from build123d import *

# Parameters (mm, degrees)
ESQUISSE1_R        = 1.5
BOSS_EXTRU_1_DEPTH = 5
BOSS_EXTRU_2_DEPTH = 20


with BuildPart() as part:
    # Esquisse1 → Boss.-Extru.1 (new body)
    with BuildSketch(Plane.XY):
        with BuildLine():
            Line((2.411392109, 3.191424149), (-33.53228234, 30.349924212))
            ThreePointArc((-33.53228234, 30.349924212), (-39.142258528, 29.531111427), (-38.389494778, 23.911891379))
            Line((-38.389494778, 23.911891379), (-2.406799918, -3.194888755))
            ThreePointArc((-2.406799918, -3.194888755), (3.193157277, -2.409096636), (2.411392109, 3.191424149))
        make_face()
        with Locations((-35.923019369, 27.102337158)):
            Circle(ESQUISSE1_R, mode=Mode.SUBTRACT)
        Circle(ESQUISSE1_R, mode=Mode.SUBTRACT)
    boss_extru_1 = extrude(amount=BOSS_EXTRU_1_DEPTH)

    # Esquisse2 → Boss.-Extru.2 (add)
    with BuildSketch(Plane(origin=(0, 0, 0), x_dir=(-1, 0, 0), z_dir=(0, 0, -1))):
        Polygon((20.560906603, 20.548947707), (25.40403733, 14.129579595), (29.397447291, 17.137928086), (24.549986024, 23.563036149), align=None)
    boss_extru_2 = extrude(amount=BOSS_EXTRU_2_DEPTH)

    # Symétrie1: Boss.-Extru.1, Boss.-Extru.2 across plane
    add(boss_extru_1.mirror(Plane.XY.offset(-20)))
    add(boss_extru_2.mirror(Plane.XY.offset(-20)))


solid = part.part
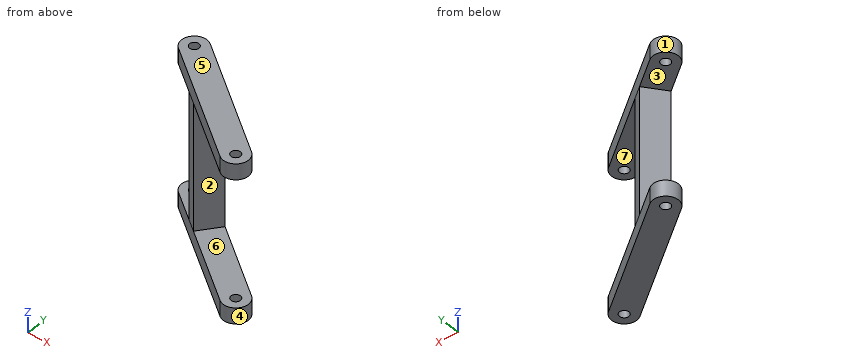
Read the model definition and answer for the solid it produces. Units are mm, in the model's axes. Face numbers are marked on the shaded views. A direction names the side the tool comes from. Coordinates: 2 decimals unless noted, no trailing zeros. Order: outer loops, then holes, each group sorted by start corner. A loop starts at its lowest first (then second) coordinate and runs counter-clockwise, first axis right, second up. Notation, with made-up numbers: (22.25, -13) -> (38.25, -13) arc R25 cw to (38.25, 9) -> close; hole circle Ø1 at (75, -40). An arc over 180 degrees is marked (long way). Answer as a JSON object with one key per item and string values.
1) Consider line 1 along Z through (x, y) = (-4, 8); line 2 along X through (y, z) = (17.5, -34.5); line 3 along Y through (x, z) = (-22.5, -39.5). Determine where each line is inside the solid, lowest interval first. Write a range as from..to.
Model answer:
{"line 1": "z = -45..-40, 0..5", "line 2": "x = -29.12..-22.86", "line 3": "y = 17.98..22.01"}
2) The mould has two halves that part along Z. Classify the marked faces 4, 5, 6 and 7: released by +Z, released by -Z, zero draft, split by the parting line, or undercut.
Model answer:
{"face 4": "zero draft", "face 5": "released by +Z", "face 6": "undercut", "face 7": "undercut"}
3) A cutting plane is placed at C-C, the plane x = -10.5. Determine the outline of the cut face in (y, z), plus the area to 3 significant figures.
Model answer:
{"outline": "(2.9, -45) -> (12.95, -45) -> (12.95, -40) -> (2.9, -40) -> close; (2.9, 0) -> (12.95, 0) -> (12.95, 5) -> (2.9, 5) -> close", "area": "100 mm²"}
4) This flat-tipped pin is pushed along its axis until it touches: pin 1 (2 mm diameter, centred on x = -29.5, z = -6, fed in from +Y). Where does it stop, or does it pass through?
Model answer:
{"pin 1": "stops at y = 18.33"}
5) A cutting plane is placed at D-D, the plane y = 4. Determine the outline of the cut face in (x, z).
Model answer:
{"outline": "(-11.96, -45) -> (1.34, -45) -> (1.34, -40) -> (-11.96, -40) -> close; (-11.96, 0) -> (1.34, 0) -> (1.34, 5) -> (-11.96, 5) -> close"}
6) A tool of negligible diameter and unlimited length cuts with its end or side. For the marked faces 1, 2 and 3, from which of +Z, -Z, +X, -X, +Y, -Y can it reach the whole face along a straight path? Write none if from no direction.
Model answer:
{"face 1": "+Z, -Z", "face 2": "+X, -Y", "face 3": "-X, +Y"}
7) A cutting plane is placed at A-A, the plane x = 0. Determine the outline of the cut face in (y, z).
Model answer:
{"outline": "(-4, -45) -> (-1.5, -45) -> (-1.5, -40) -> (-4, -40) -> close; (-4, 0) -> (-1.5, 0) -> (-1.5, 5) -> (-4, 5) -> close; (1.5, -45) -> (5.01, -45) -> (5.01, -40) -> (1.5, -40) -> close; (1.5, 0) -> (5.01, 0) -> (5.01, 5) -> (1.5, 5) -> close"}
8) A cutting plane is placed at B-B, the plane y = 0. Determine the outline of the cut face in (x, z), plus the area to 3 significant figures.
Model answer:
{"outline": "(-6.65, -45) -> (-1.5, -45) -> (-1.5, -40) -> (-6.65, -40) -> close; (-6.65, 0) -> (-1.5, 0) -> (-1.5, 5) -> (-6.65, 5) -> close; (1.5, -45) -> (4, -45) -> (4, -40) -> (1.5, -40) -> close; (1.5, 0) -> (4, 0) -> (4, 5) -> (1.5, 5) -> close", "area": "76.5 mm²"}
